from build123d import *

# Parameters (mm, degrees)
SKIZZE1_R                       = 15
SKIZZE1_R_2                     = 1.65
AUFSATZ_LINEAR_AUSTRAGEN1_DEPTH = 35.5
SKIZZE4_R                       = 2.25
SCHNITT_LINEAR_AUSTRAGEN2_DEPTH = 10
SKIZZE3_R                       = 3
SCHNITT_LINEAR_AUSTRAGEN3_DEPTH = 29.5


with BuildPart() as part:
    # Skizze1 → Aufsatz-Linear austragen1 (new body)
    with BuildSketch(Plane.XY):
        Circle(SKIZZE1_R)
        with Locations((0, -10)):
            Circle(SKIZZE1_R_2, mode=Mode.SUBTRACT)
        with Locations((-10, 0)):
            Circle(SKIZZE1_R_2, mode=Mode.SUBTRACT)
        with Locations((0, 10)):
            Circle(SKIZZE1_R_2, mode=Mode.SUBTRACT)
        with Locations((10, 0)):
            Circle(SKIZZE1_R_2, mode=Mode.SUBTRACT)
    extrude(amount=AUFSATZ_LINEAR_AUSTRAGEN1_DEPTH)

    # Skizze4 → Schnitt-Linear austragen2 (cut)
    with BuildSketch(Plane.XY.offset(35.5)):
        with Locations((7.071067812, 7.071067812)):
            Circle(SKIZZE4_R)
        with Locations((7.071067812, -7.071067812)):
            Circle(SKIZZE4_R)
        with Locations((-7.071067812, -7.071067812)):
            Circle(SKIZZE4_R)
        with Locations((-7.071067812, 7.071067812)):
            Circle(SKIZZE4_R)
    extrude(amount=-SCHNITT_LINEAR_AUSTRAGEN2_DEPTH, mode=Mode.SUBTRACT)

    # Skizze3 → Schnitt-Linear austragen3 (cut)
    with BuildSketch(Plane.XY.offset(35.5)):
        with Locations((0, 10)):
            Circle(SKIZZE3_R)
        with Locations((10, 0)):
            Circle(SKIZZE3_R)
        with Locations((0, -10)):
            Circle(SKIZZE3_R)
        with Locations((-10, 0)):
            Circle(SKIZZE3_R)
    extrude(amount=-SCHNITT_LINEAR_AUSTRAGEN3_DEPTH, mode=Mode.SUBTRACT)


solid = part.part
Verification items for the finished model (mm, model axes). A direction names the side the tool comes from. Give positions to 0.01 mm unless a question says otherwise; leave off trailing zeros. Loops run counter-clockwise (first coordinate to the right, second up) from the corner with the lowest first, then second, coordinate; pieces in that order, holes last.
1. Go/stop test with flat-tipped pins: P1, Ø1.3, axis at x = -7, y = -7.5, coming from the +Z side; P2, Ø1, axis at x = 7.5, z = 20, coming from the +Y side; P3, Ø3, axis at x = 1, y = -9, coming from the +Z side. Record where each tip stops, or that it passes through.
Derived:
P1: stops at z = 25.5
P2: stops at y = 13.27
P3: stops at z = 6
2. Cross-section at D-D on x = 11. Record the cut outline in (y, z), and give its area (3 significant figures).
Derived:
outline: (-10.2, 0) - (-1.31, 0) - (-1.31, 6) - (-2.83, 6) - (-2.83, 35.5) - (-10.2, 35.5) - close; (1.31, 0) - (10.2, 0) - (10.2, 35.5) - (2.83, 35.5) - (2.83, 6) - (1.31, 6) - close
area: 541 mm2
3. Cross-section at C-C on y = -10. Record the cut outline in (x, z).
Derived:
outline: (-11.18, 0) - (-1.65, 0) - (-1.65, 6) - (-3, 6) - (-3, 35.5) - (-11.18, 35.5) - close; (1.65, 0) - (11.18, 0) - (11.18, 35.5) - (3, 35.5) - (3, 6) - (1.65, 6) - close
4. Material ranges on probe 1 along X at (y, z) = (-0.75, 15.5); probe 2 along Z at (x, y) = (-7.5, -7); probe 3 along Y at (x, z) = (2.25, 27.5), recorded low to high.
Derived:
probe 1: x = -14.98 to -12.9, -7.1 to 7.1, 12.9 to 14.98
probe 2: z = 0 to 25.5
probe 3: y = -14.83 to -11.98, -8.02 to 8.02, 11.98 to 14.83
5. Cross-section at A-A on x = 0. Record the cut outline in (y, z), and give its area (3 significant figures).
Derived:
outline: (-15, 0) - (-11.65, 0) - (-11.65, 6) - (-13, 6) - (-13, 35.5) - (-15, 35.5) - close; (-8.35, 0) - (8.35, 0) - (8.35, 6) - (7, 6) - (7, 35.5) - (-7, 35.5) - (-7, 6) - (-8.35, 6) - close; (11.65, 0) - (15, 0) - (15, 35.5) - (13, 35.5) - (13, 6) - (11.65, 6) - close
area: 671 mm2
6. Release check for a two-part mould opening along Y. For faces 3 (the cylindrical face through (-8.857, 5.702, 30.57)), 4 (the flat face through (0, 0, 35.5)) record: +Y half, -Y half, draft (parallel to the pull), parting line (faces both ways), or undercut.
Derived:
face 3: undercut
face 4: draft
7. Tool access check on faces 1 (the flat face through (-7, -7, 25.5)), 2 (the cylindrical face through (-8.476, -0.632, 2.958)). Record the directions out of +Z, -Z, +X, -X, +Y, -Y that give a thin tool (end or side, any length) a straight path to the whole face; none if there is none.
Derived:
face 1: +Z
face 2: +Z, -Z
8. Cross-section at B-B on z = 22. Record the cut outline in (x, y).
Derived:
outline: circle Ø30 at (0, 0); hole circle Ø6 at (-10, 0); hole circle Ø6 at (0, -10); hole circle Ø6 at (0, 10); hole circle Ø6 at (10, 0)
